from build123d import *

# Parameters (mm, degrees)
SKETCH1_W           = 44.45
SKETCH1_H           = 44.45
SKETCH1_W_2         = 57
SKETCH1_H_2         = 56.4
BOSS_EXTRUDE1_DEPTH = 10
CUT_EXTRUDE1_DEPTH  = 10
CIRPATTERN1_COUNT   = 3
BOSS_EXTRUDE2_DEPTH = 10
CIRPATTERN2_COUNT   = 3
SKETCH7_W           = 30
SKETCH7_H           = 10
CUT_EXTRUDE2_DEPTH  = 10
CIRPATTERN3_COUNT   = 3
FILLET1_R           = 4
FILLET2_R           = 2


with BuildPart() as part:
    # Sketch1 → Boss-Extrude1 (new body)
    with BuildSketch(Plane(origin=(0, 82.464823413, 0), x_dir=(1, 0, 0), z_dir=(0, 1, 0))):
        with BuildLine():
            Line((-412.957473883, 60.178595798), (-412.957473883, 29.92539468))
            ThreePointArc((-412.957473883, 29.92539468), (-410.854889329, 17.127508038), (-404.768178759, 5.675053336))
            Line((-404.768178759, 5.675053336), (-277.648465327, -161.075906186))
            ThreePointArc((-277.648465327, -161.075906186), (332.742526117, 45.051995239), (-277.648465327, 251.179896664))
            Line((-277.648465327, 251.179896664), (-404.768178759, 84.428937143))
            ThreePointArc((-404.768178759, 84.428937143), (-410.854889329, 72.97648244), (-412.957473883, 60.178595798))
        make_face()
        with BuildLine():
            ThreePointArc((-234.019080144, 150.30965019), (-223.763824829, -79.948004761), (-29.482473883, -203.958143862))
            Line((-29.482473883, -203.958143862), (-29.482473883, -262.248004761))
            Line((-29.482473883, -262.248004761), (14.967526117, -262.248004761))
            Line((14.967526117, -262.248004761), (14.967526117, -203.958143862))
            ThreePointArc((14.967526117, -203.958143862), (209.248877063, -79.948004761), (219.504132378, 150.30965019))
            Line((219.504132378, 150.30965019), (269.9846327, 179.45458064))
            Line((269.9846327, 179.45458064), (247.7596327, 217.949409838))
            Line((247.7596327, 217.949409838), (197.279132378, 188.804479389))
            ThreePointArc((197.279132378, 188.804479389), (-7.257473883, 295.051995239), (-211.794080144, 188.804479389))
            Line((-211.794080144, 188.804479389), (-262.274580466, 217.949409838))
            Line((-262.274580466, 217.949409838), (-284.499580466, 179.45458064))
            Line((-284.499580466, 179.45458064), (-234.019080144, 150.30965019))
        make_face(mode=Mode.SUBTRACT)
        with Locations((-7.257473883, 342.276995239)):
            Rectangle(SKETCH1_W, SKETCH1_H, mode=Mode.SUBTRACT)
        Polygon((-272.796789122, -133.92041936), (-234.301959924, -111.69541936), (-256.526959924, -73.200590162), (-295.021789122, -95.425590162), align=None, mode=Mode.SUBTRACT)
        with Locations((-369.457473883, 45.051995239)):
            Rectangle(SKETCH1_W_2, SKETCH1_H_2, mode=Mode.SUBTRACT)
        Polygon((219.787012158, -111.69541936), (258.281841356, -133.92041936), (280.506841356, -95.425590162), (242.012012158, -73.200590162), align=None, mode=Mode.SUBTRACT)
    extrude(amount=-BOSS_EXTRUDE1_DEPTH)

    # Sketch5 → Cut-Extrude1 (cut)
    with BuildSketch(Plane(origin=(0, 82.464823413, 0), x_dir=(1, 0, 0), z_dir=(0, 1, 0))):
        Polygon((14.967526117, -239.202482577), (25.746966731, -232.248004761), (14.967526117, -232.248004761), align=None)
        Polygon((-40.261914497, -232.248004761), (-29.482473883, -232.248004761), (-29.482473883, -239.202482577), align=None)
    cut_extrude1 = extrude(amount=-CUT_EXTRUDE1_DEPTH, mode=Mode.SUBTRACT)

    # CirPattern1: Cut-Extrude1 ×3 about axis
    cirpattern1_axis = Axis((-7.257473883, 0, -45.051995239), (0, 1, 0))
    for i in range(1, CIRPATTERN1_COUNT):
        add(cut_extrude1.rotate(cirpattern1_axis, i * 360 / CIRPATTERN1_COUNT), mode=Mode.SUBTRACT)

    # Sketch6 → Boss-Extrude2 (add)
    with BuildSketch(Plane(origin=(0, 82.464823413, 0), x_dir=(1, 0, 0), z_dir=(0, 1, 0))):
        with BuildLine():
            Line((-29.482473883, -249.109608943), (-29.482473883, -270.376708747))
            Line((-29.482473883, -270.376708747), (14.967526117, -270.376708747))
            Line((14.967526117, -270.376708747), (14.967526117, -249.109608943))
            ThreePointArc((14.967526117, -249.109608943), (-7.257473883, -249.948004761), (-29.482473883, -249.109608943))
        make_face()
    boss_extrude2 = extrude(amount=-BOSS_EXTRUDE2_DEPTH)

    # CirPattern2: Boss-Extrude2 ×3 about axis
    cirpattern2_axis = Axis((-7.257473883, 72.464823413, -45.051995239), (0, 1, 0))
    for i in range(1, CIRPATTERN2_COUNT):
        add(boss_extrude2.rotate(cirpattern2_axis, i * 360 / CIRPATTERN2_COUNT))

    # Sketch7 → Cut-Extrude2 (cut)
    with BuildSketch(Plane.XZ.offset(-72.464823413)):
        with Locations((52.742526117, 227.248004761)):
            Rectangle(SKETCH7_W, SKETCH7_H)
        with Locations((-67.257473883, 227.248004761)):
            Rectangle(SKETCH7_W, SKETCH7_H)
    cut_extrude2 = extrude(amount=-CUT_EXTRUDE2_DEPTH, mode=Mode.SUBTRACT)

    # CirPattern3: Cut-Extrude2 ×3 about axis
    cirpattern3_axis = Axis((-7.257473883, 0, -45.051995239), (0, 1, 0))
    for i in range(1, CIRPATTERN3_COUNT):
        add(cut_extrude2.rotate(cirpattern3_axis, i * 360 / CIRPATTERN3_COUNT), mode=Mode.SUBTRACT)

    # Fillet1
    fillet1_edges = [part.edges().sort_by_distance(p)[0] for p in [
        (-29.482473883, 77.464823413, 239.202482577),
        (14.967526117, 77.464823413, 239.202482577),
        (250.026625045, 77.464823413, -167.931819548),
        (227.801625045, 77.464823413, -206.426648746),
        (-242.316572811, 77.464823413, -206.426648746),
        (-264.541572811, 77.464823413, -167.931819548),
        (14.967526117, 77.464823413, 249.109608943),
        (-29.482473883, 77.464823413, 249.109608943),
        (258.606448157, 77.464823413, -172.885382731),
        (236.381448157, 77.464823413, -211.380211929),
        (-273.121395923, 77.464823413, -172.885382731),
        (-250.896395923, 77.464823413, -211.380211929),
        (-29.482473883, 77.464823413, 203.958143862),
        (14.967526117, 77.464823413, 203.958143862),
        (219.504132378, 77.464823413, -150.30965019),
        (197.279132378, 77.464823413, -188.804479389),
        (-211.794080144, 77.464823413, -188.804479389),
        (-234.019080144, 77.464823413, -150.30965019),
    ]]
    fillet(fillet1_edges, radius=FILLET1_R)

    # Fillet2
    fillet2_edges = [part.edges().sort_by_distance(p)[0] for p in [
        (-397.957473883, 77.464823413, -73.251995239),
        (-397.957473883, 77.464823413, -16.851995239),
        (-340.957473883, 77.464823413, -16.851995239),
        (-340.957473883, 77.464823413, -73.251995239),
    ]]
    fillet(fillet2_edges, radius=FILLET2_R)


solid = part.part
Read the model definition and answer for the solid it produces. Units are mm, in the model's axes. A direction names the side the tool comes from. Round coordinates to 2 decimals unless told otherwise and drop trailing zeros. Loops run counter-clockwise (first coordinate to the right, second up) from the corner with the lowest first, then second, coordinate; pieces in that order, holes last.
Q1. Each of these flat-tipped pins is pushed along its axis until it touches: pin 1 (3 mm diameter, centred on x = -372.5, y = 76.5, fed in from +Z); pin 2 (5 mm diameter, centred on x = -68, y = 75.5, fed in from +Z); pin 3 (5 mm diameter, centred on x = 18.5, y = 76, fed in from +Z). Where does it stop, or does it pass through?
Q2. Section A-A on z = -276 is taken. Write down the section's boundary in (x, y).
Q3. Consider probe 1 along X at (y, z) = (79.5, -70); probe 2 along Z at (x, y) = (221.5, 77.25); probe 3 along X at (y, z) = (79.75, 99.5). Determine where each line is inside the solid, lowest interval first.
Q4. Section D-D on z = -52 is taken. Write down the section's boundary in (x, y), and give its area (3 significant figures).
Q5. Section B-B on x = -121 is taken. Write down the section's boundary in (y, z).
Q6. Which of the six approach directions +Z, -Z, +X, -X, +Y, -Y give full straight-line access (tool end or side, diameter ignored) to faces 5 (the face through (-262.864, 77.535, -192.328)), 6 (the face through (-141.5, 82.465, 166.4))?
Q7. Section C-C on z = -129.5 is taken. Write down the section's boundary in (x, y), and give its area (3 significant figures).
Q8. Determine the mould class of faces 1 (the face through (-340.32, 77.53, -168.97)), 2 (the face through (207.578, 77.535, 82.798)), 3 (the face through (-284.065, 77.535, 114.404)), 4 (the face through (332.536, 77.535, -33.201)) for opening direction X: released by +X, released by -X, zero draft, split by the parting line, or undercut.
Output:
1. pin 1: stops at z = 38.62
1. pin 2: stops at z = 289.92
1. pin 3: stops at z = 294.15
2. outline: (-256.78, 72.46) - (-102.98, 72.46) - (-102.98, 82.46) - (-256.78, 82.46) - close; (88.47, 72.46) - (242.27, 72.46) - (242.27, 82.46) - (88.47, 82.46) - close
3. probe 1: x = -411.73 to -397.96, -340.96 to -256.01, 241.49 to 331.83
3. probe 2: z = -296.59 to -209.66, -203.43 to -202.79, -151.13 to -145.9, 55.79 to 108.73, 112.68 to 206.48
3. probe 3: x = -324.59 to -292.67, -241.34 to -211.23, 196.71 to 226.83, 278.15 to 300.48
4. outline: (-412.96, 72.46) - (-397.96, 72.46) - (-397.96, 82.46) - (-412.96, 82.46) - close; (-340.96, 72.46) - (-257.16, 72.46) - (-257.16, 82.46) - (-340.96, 82.46) - close; (242.65, 72.46) - (332.67, 72.46) - (332.67, 82.46) - (242.65, 82.46) - close
4. area: 1,890 mm2
5. outline: (72.46, -365.46) - (82.46, -365.46) - (82.46, -267.68) - (72.46, -267.68) - close; (72.46, 177.57) - (82.46, 177.57) - (82.46, 275.36) - (72.46, 275.36) - close
6. face 5: +Y, -Y
6. face 6: +Z, -Z, +X, -X, +Y
7. outline: (-370.41, 72.46) - (-278.7, 72.46) - (-278.7, 82.46) - (-370.41, 82.46) - close; (-267.15, 72.46) - (-242.56, 72.46) - (-242.56, 82.46) - (-267.15, 82.46) - close; (228.05, 72.46) - (252.64, 72.46) - (252.64, 82.46) - (228.05, 82.46) - close; (264.18, 72.46) - (322.09, 72.46) - (322.09, 82.46) - (264.18, 82.46) - close
7. area: 1,990 mm2
8. face 1: released by -X
8. face 2: undercut
8. face 3: undercut
8. face 4: split by the parting line
